from build123d import *

# Parameters (mm, degrees)
SKETCH1_R           = 4.75
BOSS_EXTRUDE1_DEPTH = 0.0001
BOSS_EXTRUDE2_START = 105
SKETCH4_R           = 4.75
BOSS_EXTRUDE2_DEPTH = 105
CUT_EXTRUDE3_DEPTH  = 4
SKETCH6_R           = 4.75
CUT_EXTRUDE4_DEPTH  = 5


with BuildPart() as part:
    # Sketch1 → Boss-Extrude1 (new body)
    with BuildSketch(Plane.XY):
        Circle(SKETCH1_R)
    extrude(amount=BOSS_EXTRUDE1_DEPTH)

    # Sketch4 → Boss-Extrude2 (add)
    with BuildSketch(Plane(origin=(0, 0, 0), x_dir=(-1, 0, 0), z_dir=(0, 0, -1)).offset(BOSS_EXTRUDE2_START)):
        Circle(SKETCH4_R)
    extrude(amount=-BOSS_EXTRUDE2_DEPTH)

    # Sketch5 → Cut-Extrude3 (cut)
    with BuildSketch(Plane(origin=(0, 4.75, 0), x_dir=(1, 0, 0), z_dir=(0, 1, 0))):
        with BuildLine():
            Line((-2, 10), (-2, 20))
            ThreePointArc((-2, 20), (0, 22), (2, 20))
            Line((2, 20), (2, 10))
            ThreePointArc((2, 10), (0, 8), (-2, 10))
        make_face()
        with BuildLine():
            Line((-2, 50), (-2, 58.71))
            ThreePointArc((-2, 58.71), (0, 60.71), (2, 58.71))
            Line((2, 58.71), (2, 50))
            ThreePointArc((2, 50), (0, 48), (-2, 50))
        make_face()
        with BuildLine():
            Line((-2, 69.62), (-2, 74.62))
            ThreePointArc((-2, 74.62), (0, 76.62), (2, 74.62))
            Line((2, 74.62), (2, 69.62))
            ThreePointArc((2, 69.62), (0, 67.62), (-2, 69.62))
        make_face()
    extrude(amount=-CUT_EXTRUDE3_DEPTH, mode=Mode.SUBTRACT)

    # Sketch6 → Cut-Extrude4 (cut)
    with BuildSketch(Plane(origin=(0, 0, -105), x_dir=(-1, 0, 0), z_dir=(0, 0, -1))):
        Circle(SKETCH6_R)
    extrude(amount=-CUT_EXTRUDE4_DEPTH, mode=Mode.SUBTRACT)


solid = part.part
Could you check a few things on this model? Use its own coordinates, in mm. Coordinates: 2 decimals unless noted, no trailing zeros. Loops run counter-clockwise (first coordinate to the right, second up) from the corner with the lowest first, then second, coordinate; pieces in that order, holes last. Notation, with made-up numbers: (-14.75, 61) -> (18.25, 61) arc R20 ccw to (18.25, 92) -> close; hole circle Ø10 at (1.5, 81.25). An arc over 180 degrees is marked (long way). Answer in a Markdown table with one row per item.
(1) Thinking about a two-plate mould opening in Z: for faces 1 (the face through (-0.04, 2.78, -60.71)), 2 (the face through (0, 0, -100)), 3 (the face through (0, 0, 0)), which applies, released by +Z, released by -Z, zero draft, split by the parting line, or undercut?
Results found:
| item | result |
|---|---|
| face 1 | undercut |
| face 2 | released by -Z |
| face 3 | released by +Z |
(2) Imagine slicing it at A-A (x = 0). List the corners of the cut face in (y, z) for me.
Results found:
| item | result |
|---|---|
| outline | (-4.75, -100) -> (4.75, -100) -> (4.75, -76.62) -> (0.75, -76.62) -> (0.75, -67.62) -> (4.75, -67.62) -> (4.75, -60.71) -> (0.75, -60.71) -> (0.75, -48) -> (4.75, -48) -> (4.75, -22) -> (0.75, -22) -> (0.75, -8) -> (4.75, -8) -> (4.75, 0) -> (-4.75, 0) -> close |
(3) Imagine slicing it at B-B (y = 2.75). List the corners of the cut face in (x, z) for me.
Results found:
| item | result |
|---|---|
| outline | (-3.87, -100) -> (3.87, -100) -> (3.87, 0) -> (-3.87, 0) -> close; hole (-2, -74.62) arc R2 ccw to (2, -74.62) -> (2, -69.62) arc R2 ccw to (-2, -69.62) -> close; hole (-2, -58.71) arc R2 ccw to (2, -58.71) -> (2, -50) arc R2 ccw to (-2, -50) -> close; hole (-2, -20) arc R2 ccw to (2, -20) -> (2, -10) arc R2 ccw to (-2, -10) -> close |
(4) Will these pins go through, and if not, where does the flat tip stop? pin 1 Ø3 at (y, z) = (2.5, -71.5) entering from +X; pin 2 Ø5 at (x, z) = (-2, -40) entering from +Y; pin 3 Ø3 at (y, z) = (2.5, -13.5) entering from -X; pin 4 Ø1.1 at (y, z) = (2.5, -71) entering from -X.
Results found:
| item | result |
|---|---|
| pin 1 | stops at x = 4.64 |
| pin 2 | stops at y = 4.75 |
| pin 3 | stops at x = -4.64 |
| pin 4 | stops at x = -4.33 |
(5) If I drill on probe 1 along Z at (x, y) = (1, 2.75); probe 2 along Z at (x, y) = (1.5, 2.5); probe 3 along X at (y, z) = (2.75, -49), over which ranges is the centre line in solid material (lowest first)?
Results found:
| item | result |
|---|---|
| probe 1 | z = -100 to -76.35, -67.89 to -60.44, -48.27 to -21.73, -8.27 to 0 |
| probe 2 | z = -100 to -75.94, -68.3 to -60.03, -48.68 to -21.32, -8.68 to 0 |
| probe 3 | x = -3.87 to -1.73, 1.73 to 3.87 |
(6) Imagine slicing it at D-D (y = -2.25). List the corners of the cut face in (x, z) for me, plus the area to 3 significant figures.
Results found:
| item | result |
|---|---|
| outline | (-4.18, -100) -> (4.18, -100) -> (4.18, 0) -> (-4.18, 0) -> close |
| area | 837 mm^2 |
(7) Imagine slicing it at C-C (z = -11.5). List the corners of the cut face in (x, y) for me, plus the area to 3 significant figures.
Results found:
| item | result |
|---|---|
| outline | (-2, 0.75) -> (-2, 4.31) arc R4.75 ccw (long way) to (2, 4.31) -> (2, 0.75) -> close |
| area | 55.5 mm^2 |
